For this review, use the dimensioned drawing (mm, ordinates from the lowest corner) and the shaded views. A direction names the side the tool comes from. Round coordinates to 2 decimals unless told otherwise and drop trailing zeros. Loops run counter-clockwise (first coordinate to the right, second up) from the corner with the lowest first, then second, coordinate; pieces in that order, holes last. Notation, with made-up numbers: M 55,-30 L 100,-30 A14 cw 100,-17 Z; hole C 47,-14.75 d6. An arc over 180 degrees is marked long. One line per item, written item: value. Start each with the question number.
Item 1: We need section A-A (x = 10.16). Write out the cut boundary in (y, z).
Item 2: Clearance check with flat-ended pins moving along their axes: pin 1 (2.5 mm diameter, centred on x = 10, z = 17, fed in from +Y); pin 2 (4.5 mm diameter, centred on x = 21, y = 4.5, fed in from +Z); pin 3 (4 mm diameter, centred on y = 3, z = 27, fed in from +X). State where each tip first meets the part, or that it passes through.
Item 3: We need section C-C (y = 5). Write out the cut boundary in (x, z), then the cut area to 3 significant figures.
Item 4: Mouldability with a two-part tool opening along X and no side actions: class the marked faces 3, 4 and 5 as released by +X, released by -X, zero draft, split by the parting line, or undercut.
Item 5: For line 1 along Z through (x, y) = (10.16, 4.25); line 2 along X through (y, z) = (7.25, 9) (3 decimals); line 3 along Y through (x, z) = (20.32, 22.7), list the stretches that pass through material, from the lowest coordinate up.
Item 6: For the marked faces 1 and 2, list the 3-axis set-ups (+Z, -Z, +X, -X, +Y, -Y) from which the entire face can be reached by the end or side of a thin tool; tool diameter is ignored.
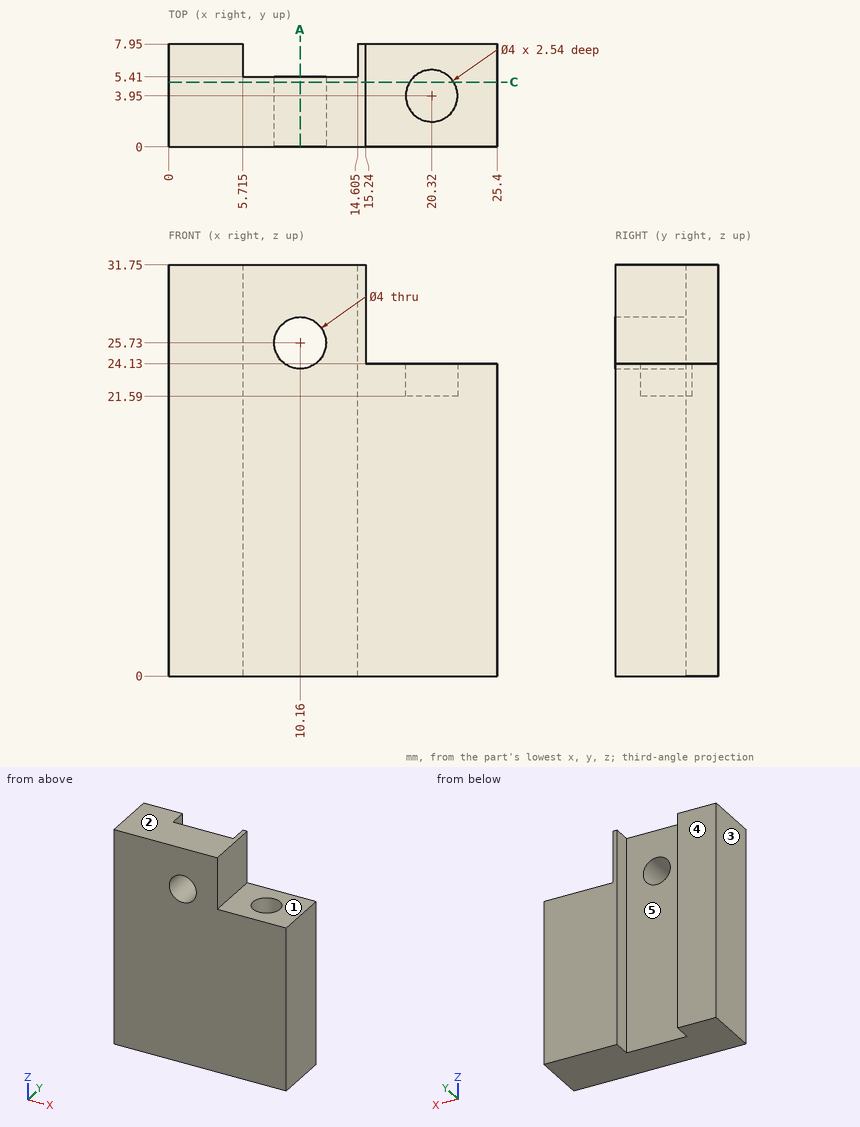
A:
1. outline: M 0,0 L 5.41,0 L 5.41,23.73 L 0,23.73 Z; M 0,27.73 L 5.41,27.73 L 5.41,31.75 L 0,31.75 Z
2. pin 1: y = 5.41
2. pin 2: z = 24.13
2. pin 3: x = 15.24
3. outline: M 0,0 L 25.4,0 L 25.4,24.13 L 22.02,24.13 L 22.02,21.59 L 18.62,21.59 L 18.62,24.13 L 15.24,24.13 L 15.24,31.75 L 0,31.75 Z; hole C 10.16,25.73 d4
3. area: 708 mm2
4. face 3: released by -X
4. face 4: zero draft
4. face 5: undercut
5. line 1: 0 to 23.73, 27.73 to 31.75
5. line 2: 0 to 5.715, 14.605 to 25.4
5. line 3: 0 to 1.95, 5.95 to 7.95
6. face 1: +Z, +X, +Y, -Y
6. face 2: +Z, +X, -X, +Y, -Y
